from build123d import *

# Parameters (mm, degrees)
F1_DEPTH = 1.7
F3_DEPTH = 1.6


with BuildPart() as f1:
    # F0 (on Top) → F1 (new body)
    with BuildSketch(Plane.XY):
        with BuildLine():
            Line((-4.5, -16), (4.5, -16))
            ThreePointArc((4.5, -16), (12.5, -24), (20.5, -16))
            Line((20.5, -16), (20.5, -5.5))
            Line((20.5, -5.5), (-20.5, -5.5))
            Line((-20.5, -5.5), (-20.5, -16))
            ThreePointArc((-20.5, -16), (-12.5, -24), (-4.5, -16))
        make_face()
    extrude(amount=F1_DEPTH)


with BuildPart() as f3:
    # F2 (on Top) → F3 (new body)
    with BuildSketch(Plane.XY):
        Polygon((28, 0), (0, 0), (-28, 0), (-28, -30), (28, -30), align=None)
    extrude(amount=F3_DEPTH)

    # F4: cut F1
    add(f1.part, mode=Mode.SUBTRACT)


solid = f3.part
Geometry check sheet. Reference: the model listing, model coordinates, mm. A direction names the side the tool comes from. Coordinates: 2 decimals unless noted, no trailing zeros. Order: outer loops, then holes, each group sorted by start corner. A loop starts at its lowest first (then second) coordinate and runs counter-clockwise, first axis right, second up. Notation, with made-up numbers: (-13.75, 45.25) -> (-9.75, 45.25) arc R28 cw to (-9.75, 71.25) -> close; hole circle Ø1 at (45.25, 23). An arc over 180 degrees is marked (long way). Use a Markdown table: item, result. Add a question column.
1. Cross-section at C-C (z = 0.75). Enter the section's corners in (x, y), and give its area (3 significant figures).
2. Cross-section at A-A (y = -15). Enter the section's corners in (x, z), and give its area (3 significant figures).
3. Cross-section at B-B (x = -1.5). Enter the section's corners in (y, z), and give its area (3 significant figures).
4. Material ranges on L1, parallel to X at y = -9.5, z = 0.75; L2, parallel to Y at x = -14.5, z = 0.4; L3, parallel to Y at x = 7.5, z = 0.2 (3 decimals), recorded low to high.
5. Cross-section at D-D (y = -19). Enter the section's corners in (x, z), and give its area (3 significant figures).
6. Mould release check, pull along X, two halves, no side actions. Record for faces 1 (the face through (-12.676, -23.998, 0.789)), 2 (the face through (0, -18, 1.6)), 3 (the face through (-28, -15, 1)): pulls with the +X half, pulls with the -X half, needs draft (parallel to the pull), parting line crosses it, or undercut.
7. Set-up check for faces 4 (the face through (0, -5.5, 1)), 5 (the face through (0, -30, 1)): record each of +Z, -Z, +X, -X, +Y, -Y from which the full face is reachable in a straight line by a thin tool's end or side.
Filled sheet:
| question | item | result |
|---|---|---|
| 1 | outline | (-28, -30) -> (28, -30) -> (28, 0) -> (-28, 0) -> close; hole (-20.5, -16) arc R8 ccw to (-4.5, -16) -> (4.5, -16) arc R8 ccw to (20.5, -16) -> (20.5, -5.5) -> (-20.5, -5.5) -> close |
| 1 | area | 1,050 mm2 |
| 2 | outline | (-28, 0) -> (-20.5, 0) -> (-20.5, 1.6) -> (-28, 1.6) -> close; (20.5, 0) -> (28, 0) -> (28, 1.6) -> (20.5, 1.6) -> close |
| 2 | area | 24.0 mm2 |
| 3 | outline | (-30, 0) -> (-16, 0) -> (-16, 1.6) -> (-30, 1.6) -> close; (-5.5, 0) -> (0, 0) -> (0, 1.6) -> (-5.5, 1.6) -> close |
| 3 | area | 31.2 mm2 |
| 4 | L1 | -28 to -20.5, 20.5 to 28 |
| 4 | L2 | -30 to -23.75, -5.5 to 0 |
| 4 | L3 | -30 to -22.245, -5.5 to 0 |
| 5 | outline | (-28, 0) -> (-19.92, 0) -> (-19.92, 1.6) -> (-28, 1.6) -> close; (-5.08, 0) -> (5.08, 0) -> (5.08, 1.6) -> (-5.08, 1.6) -> close; (19.92, 0) -> (28, 0) -> (28, 1.6) -> (19.92, 1.6) -> close |
| 5 | area | 42.1 mm2 |
| 6 | face 1 | undercut |
| 6 | face 2 | needs draft |
| 6 | face 3 | pulls with the -X half |
| 7 | face 4 | +Z, -Z |
| 7 | face 5 | +Z, -Z, +X, -X, -Y |
